Verification items for this drawing (mm, ordinates from the low corner). Round coordinates to 2 decimals unless told otherwise and drop trailing zeros. Order: outer loops, then holes, each group sorted by start corner. A loop starts at its lowest first (then second) coordinate and runs counter-clockwise, first axis right, second up. Notation, with made-up numbers: (29, -24) -> (85, -24) arc R21 cw to (85, -9) -> close; hole circle Ø2 at (7.25, 73.25). An arc over 180 degrees is marked (long way). Answer in a Markdown table with one row per item.
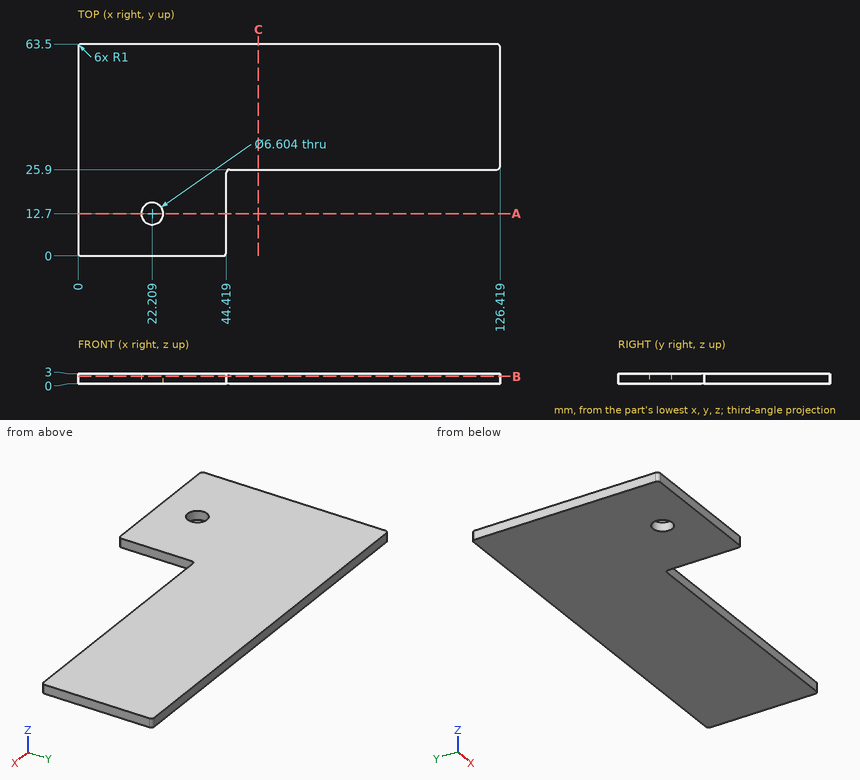
Item 1: Cross-section at A-A (y = 12.7). Record the boundary of the cut face in (x, z).
Result sheet:
| item | result |
|---|---|
| outline | (0, 0) -> (18.91, 0) -> (18.91, 3) -> (0, 3) -> close; (25.51, 0) -> (44.42, 0) -> (44.42, 3) -> (25.51, 3) -> close |
Item 2: Cross-section at B-B (z = 2.25). Record the boundary of the cut face in (x, y).
Result sheet:
| item | result |
|---|---|
| outline | (0, 1) arc R1 ccw to (1, 0) -> (43.42, 0) arc R1 ccw to (44.42, 1) -> (44.42, 24.9) arc R1 cw to (45.42, 25.9) -> (125.42, 25.9) arc R1 ccw to (126.42, 26.9) -> (126.42, 62.5) arc R1 ccw to (125.42, 63.5) -> (1, 63.5) arc R1 ccw to (0, 62.5) -> close; hole circle Ø6.6 at (22.21, 12.7) |
Item 3: Cross-section at C-C (x = 54). Record the boundary of the cut face in (y, z), and give its area (3 significant figures).
Result sheet:
| item | result |
|---|---|
| outline | (25.9, 0) -> (63.5, 0) -> (63.5, 3) -> (25.9, 3) -> close |
| area | 113 mm^2 |
Item 4: Scan lines: line 1 (Y direction, x = 83, z = 1.2); line 2 (X direction, y = 22, z = 1.3); line 3 (Y direction, x = 44, z = 1.7) (1 decimal). Record each from-to range of solid material in increasing order. Write a range as [from, to].
Result sheet:
| item | result |
|---|---|
| line 1 | y = [25.9, 63.5] |
| line 2 | x = [0, 44.42] |
| line 3 | y = [0.2, 63.5] |
Item 5: Depth check by flat-ended pin: P1, Ø12, axis at x = 84, y = 33, coming from the -Z side. Enter the tip coordinate at first touch or a pass-through.
Result sheet:
| item | result |
|---|---|
| P1 | stops at z = 0 |
